Geometry check sheet. Reference: the model listing, model coordinates, mm. A direction names the side the tool comes from. Give positions to 0.01 mm unless a question says otherwise; leave off trailing zeros. Order: outer loops, then holes, each group sorted by start corner. A loop starts at its lowest first (then second) coordinate and runs counter-clockwise, first axis right, second up.
from build123d import *

# Parameters (mm, degrees)
F0_W     = 145
F0_H     = 106.5
F0_W_2   = 106
F0_H_2   = 44
F0_R     = 5
F1_DEPTH = 5
F2_SIZE2 = 8.5
F2_SIZE  = 4
F4_DEPTH = 3


with BuildPart() as f1:
    # F0 (on Front) → F1 (new body)
    with BuildSketch(Plane.XZ):
        with Locations((72.5, 53.25)):
            Rectangle(F0_W, F0_H)
        with Locations((70, 44)):
            Rectangle(F0_W_2, F0_H_2, mode=Mode.SUBTRACT)
        with BuildLine():
            ThreePointArc((26, 82), (26.585786, 83.414214), (28, 84))
            Line((28, 84), (43, 84))
            ThreePointArc((43, 84), (44.414214, 83.414214), (45, 82))
            Line((45, 82), (45, 74))
            ThreePointArc((45, 74), (44.414214, 72.585786), (43, 72))
            Line((43, 72), (28, 72))
            ThreePointArc((28, 72), (26.585786, 72.585786), (26, 74))
            Line((26, 74), (26, 82))
        make_face(mode=Mode.SUBTRACT)
        with Locations((58, 95.5)):
            Circle(F0_R, mode=Mode.SUBTRACT)
        with BuildLine():
            Line((87, 100.5), (98, 100.5))
            ThreePointArc((98, 100.5), (101.535534, 99.035534), (103, 95.5))
            ThreePointArc((103, 95.5), (101.535534, 91.964466), (98, 90.5))
            Line((98, 90.5), (87, 90.5))
            ThreePointArc((87, 90.5), (83.464466, 91.964466), (82, 95.5))
            ThreePointArc((82, 95.5), (83.464466, 99.035534), (87, 100.5))
        make_face(mode=Mode.SUBTRACT)
    extrude(amount=-F1_DEPTH)

    # F2
    f2_edges = [f1.edges().sort_by_distance(p)[0] for p in [
        (17, 0, 44),
    ]]
    chamfer(f2_edges, length=F2_SIZE, length2=F2_SIZE2)

    # F3 (on face) → F4 (join)
    with BuildSketch(Plane(origin=(0, 5, 0), x_dir=(-1, 0, 0), z_dir=(0, 1, 0))):
        Polygon((-123, 66), (-17, 66), (-17, 69), (-126, 69), (-126, 19), (-17, 19), (-17, 22), (-123, 22), align=None)
    extrude(amount=F4_DEPTH)


solid = f1.part
Item 1: Scan lines: L1, parallel to Z at x = 58, y = 1.45; L2, parallel to Z at x = 85.5, y = 3.25; L3, parallel to X at y = 6, z = 64. Record each from-to range of solid material in increasing order.
Reported:
L1: z = 0 to 22, 66 to 90.5, 100.5 to 106.5
L2: z = 0 to 22, 66 to 90.73, 100.27 to 106.5
L3: x = 123 to 126
Item 2: Sectioned sample at A-A (x = 58). Enter the section's corners in (y, z), and give its area (4 significant figures).
Reported:
outline: (0, 0) - (5, 0) - (5, 19) - (8, 19) - (8, 22) - (0, 22) - close; (0, 66) - (8, 66) - (8, 69) - (5, 69) - (5, 90.5) - (0, 90.5) - close; (0, 100.5) - (5, 100.5) - (5, 106.5) - (0, 106.5) - close
area: 280.5 mm2
Item 3: Set-up check for faces 1 (the flat face through (12.69, 1.97, 43.69)), 2 (the flat face through (71, 6, 69)), 3 (the flat face through (17, 6, 20)), 4 (the flat face through (45, 2, 78)): record each of +Z, -Z, +X, -X, +Y, -Y from which the full face is reachable in a straight line by a thin tool's end or side.
Reported:
face 1: -Y
face 2: +Z, +X, -X, +Y
face 3: +Z, -Z, -X, +Y
face 4: +Y, -Y
Item 4: Draft check along X on faces 5 (the flat face through (83.9, 8, 66.3)), 6 (the flat face through (0, 2, 53)), 7 (the flat face through (67, 4, 66)), 8 (the flat face through (126, 6, 44)). Enter one of: released by +X, released by -X, zero draft, split by the parting line, or undercut.
Reported:
face 5: zero draft
face 6: released by -X
face 7: undercut
face 8: released by +X
Item 5: Sectioned sample at B-B (z = 29.5). Enter the section's corners in (x, y).
Reported:
outline: (0, 0) - (8.5, 0) - (17, 4) - (17, 5) - (0, 5) - close; (123, 0) - (145, 0) - (145, 5) - (126, 5) - (126, 8) - (123, 8) - close
Item 6: Sectioned sample at C-C (x = 76.5). Enter the section's corners in (y, z).
Reported:
outline: (0, 0) - (5, 0) - (5, 19) - (8, 19) - (8, 22) - (0, 22) - close; (0, 66) - (8, 66) - (8, 69) - (5, 69) - (5, 106.5) - (0, 106.5) - close
Item 7: Sectioned sample at D-D (y = 1.25). Enter the section's corners in (x, z).
Reported:
outline: (0, 0) - (145, 0) - (145, 106.5) - (0, 106.5) - close; hole (11.16, 22) - (123, 22) - (123, 66) - (11.16, 66) - close; hole (26, 74) arc R2 ccw to (28, 72) - (43, 72) arc R2 ccw to (45, 74) - (45, 82) arc R2 ccw to (43, 84) - (28, 84) arc R2 ccw to (26, 82) - close; hole circle Ø10 at (58, 95.5); hole (87, 90.5) - (98, 90.5) arc R5 ccw to (98, 100.5) - (87, 100.5) arc R5 ccw to start
Item 8: Gauge pin test, flat ends, axial feed: pin 1 (1.5 mm diameter, centred on x = 48, y = 6.5, fed in from +Z); pin 2 (2.5 mm diameter, centred on y = 6.5, z = 20.5, fed in from -X); pin 3 (1.5 mm diameter, centred on x = 85.5, y = 6.5, fed in from -Z). Record the tip position at first contact, or that the pin passes through.
Reported:
pin 1: stops at z = 69
pin 2: stops at x = 17
pin 3: stops at z = 19
